```python
from build123d import *

# Parameters (mm, degrees)
SKETCH1_R           = 4
BOSS_EXTRUDE1_DEPTH = 14
SKETCH2_R           = 2.75
CUT_EXTRUDE1_DEPTH  = 6
SKETCH3_W           = 2
SKETCH3_H           = 11.620769134
CUT_EXTRUDE2_DEPTH  = 14
SKETCH4_R           = 2
CUT_EXTRUDE3_DEPTH  = 9
SKETCH5_R           = 3.5
CUT_EXTRUDE4_DEPTH  = 4
SKETCH6_R           = 1.85
CUT_EXTRUDE5_DEPTH  = 9
FILLET1_R           = 0.3


with BuildPart() as part:
    # Sketch1 → Boss-Extrude1 (new body)
    with BuildSketch(Plane.XY):
        Polygon((-20.938905162, 0.786403392), (-8.938905162, 0.786403392), (-8.938905162, 27.286403392), (8.761094838, 27.286403392), (8.761094838, 0.786403392), (20.761094838, 0.786403392), (20.761094838, -4.713596608), (-20.938905162, -4.713596608), align=None)
        with Locations((0, 15.286403392)):
            Circle(SKETCH1_R, mode=Mode.SUBTRACT)
    extrude(amount=BOSS_EXTRUDE1_DEPTH)

    # Sketch2 → Cut-Extrude1 (cut)
    with BuildSketch(Plane(origin=(0, 0.786403392, 0), x_dir=(1, 0, 0), z_dir=(0, 1, 0))):
        with Locations((-15.9, -7)):
            Circle(SKETCH2_R)
        with Locations((15.9, -7)):
            Circle(SKETCH2_R)
    extrude(amount=-CUT_EXTRUDE1_DEPTH, mode=Mode.SUBTRACT)

    # Sketch3 → Cut-Extrude2 (cut)
    with BuildSketch(Plane.XY.offset(14)):
        with Locations((0.152630001, 23.872597077)):
            Rectangle(SKETCH3_W, SKETCH3_H)
    extrude(amount=-CUT_EXTRUDE2_DEPTH, mode=Mode.SUBTRACT)

    # Sketch4 → Cut-Extrude3 (cut)
    with BuildSketch(Plane(origin=(8.761094838, 0, 0), x_dir=(0, 0, -1), z_dir=(1, 0, 0))):
        with Locations((-7, 22.786403392)):
            Circle(SKETCH4_R)
    extrude(amount=-CUT_EXTRUDE3_DEPTH, mode=Mode.SUBTRACT)

    # Sketch5 → Cut-Extrude4 (cut)
    with BuildSketch(Plane(origin=(8.761094838, 0, 0), x_dir=(0, 0, -1), z_dir=(1, 0, 0))):
        with Locations((-7, 22.786403392)):
            Circle(SKETCH5_R)
    extrude(amount=-CUT_EXTRUDE4_DEPTH, mode=Mode.SUBTRACT)

    # Sketch6 → Cut-Extrude5 (cut)
    with BuildSketch(Plane.ZY.offset(8.938905162)):
        with Locations((7, 22.786403392)):
            Circle(SKETCH6_R)
    extrude(amount=-CUT_EXTRUDE5_DEPTH, mode=Mode.SUBTRACT)

    # Fillet1
    fillet1_edges = [part.edges().sort_by_distance(p)[0] for p in [
        (-20.938905162, 0.786403392, 7),
        (-8.938905162, 27.286403392, 7),
        (8.761094838, 27.286403392, 7),
        (20.761094838, 0.786403392, 7),
    ]]
    fillet(fillet1_edges, radius=FILLET1_R)


solid = part.part
```
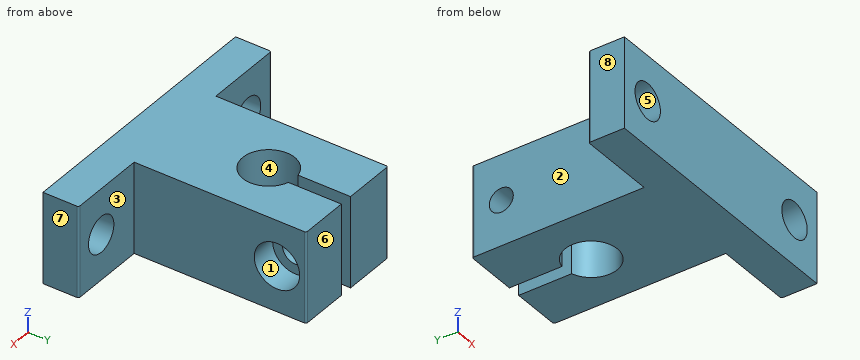
The listing builds one solid part. Answer for the finished solid, in the listing's coordinates (mm). Face numbers are marked on the shaded views. A direction names the side the tool comes from. Round coordinates to 2 decimals unless told otherwise and drop trailing zeros. Loops run counter-clockwise (first coordinate to the right, second up) from the corner with the lowest first, then second, coordinate; pieces in that order, holes last. Notation, with made-up numbers: (11, 6.5) - (53, 6.5) arc R21 cw to (53, 18.5) - close; hole circle Ø3 at (8.5, 21). An arc over 180 degrees is marked (long way). Return JSON: item names as keys, results as strings. Group by question number.
1. Consider probe 1 along X at (y, z) = (-1.65, 7); probe 2 along Y at (x, z) = (7.4, 7); probe 3 along Y at (x, z) = (-3, 7). Determine where each line is inside the solid, lowest interval first.
2. The part is cut by section B-B on x = -15.9. Determine the outline of the cut face in (y, z).
3. Each of these flat-tipped pins is pushed along its axis until it touches: P1, Ø6, axis at y = 13, z = 5.5, coming from the +X side; P2, Ø2, axis at y = 22.79, z = 7, coming from the -X side; P3, Ø8, axis at y = 23.5, z = 8.5, coming from the -X side; P4, Ø6.5, axis at y = 22.79, z = 7, coming from the +X side. Where does it stop, or does it pass through?
4. The part is cut by section A-A on x = -2. Determine the outline of the cut face in (y, z), then the cut area to 3 significant figures.
5. Which of the six approach directions +Z, -Z, +X, -X, +Y, -Y give full straight-line access (tool end or side, diameter ignored) to the marked faces 1, 2, 3 and 4?
6. The part is cut by section D-D on z = 7. State how many separate pieces and enclosed holes the cut face has, then the cut area to 3 significant figures.
7. The part is cut by section C-C on y = 16. Determine the outline of the cut face in (x, z), then the cut area to 3 significant figures.
8. The mould has two halves that part along X. Classify the marked faces 5, 6, 7 and 8: pulls with the +X half, pulls with the -X half, needs draft (parallel to the pull), parting line crosses it, or undercut.
Resolved:
{
 "1": {"probe 1": "x = -20.94 to -18.65, -13.15 to 13.15, 18.65 to 20.76", "probe 2": "y = -4.71 to 19.29, 26.29 to 27.29", "probe 3": "y = -4.71 to 12.64, 17.93 to 20.94, 24.64 to 27.29"},
 "2": {"outline": "(-4.71, 0) - (0.79, 0) - (0.79, 4.25) - (-4.71, 4.25) - close; (-4.71, 9.75) - (0.79, 9.75) - (0.79, 14) - (-4.71, 14) - close"},
 "3": {"P1": "stops at x = 8.76", "P2": "passes through", "P3": "stops at x = -8.94", "P4": "stops at x = 4.76"},
 "4": {"outline": "(-4.71, 0) - (11.82, 0) - (11.82, 14) - (-4.71, 14) - close; (18.75, 0) - (27.29, 0) - (27.29, 14) - (18.75, 14) - close; hole circle Ø3.7 at (22.79, 7)", "area": "340 mm²"},
 "5": {"face 1": "+X", "face 2": "+Z, -Z, -X, +Y", "face 3": "+Z, -Z, +X, +Y", "face 4": "+Z, -Z"},
 "6": {"separate pieces": "5", "enclosed holes": "0", "area": "499 mm²"},
 "7": {"outline": "(-8.94, 0) - (-3.94, 0) - (-3.94, 14) - (-8.94, 14) - close; (3.94, 0) - (8.76, 0) - (8.76, 14) - (3.94, 14) - close", "area": "138 mm²"},
 "8": {"face 5": "undercut", "face 6": "needs draft", "face 7": "pulls with the +X half", "face 8": "pulls with the -X half"}
}
